Could you check a few things on this drawing? It's one solid part, dimensions in mm from its lowest x, y, z. A direction names the side the tool comes from. Round coordinates to 2 decimals unless told otherwise and drop trailing zeros. Loops run counter-clockwise (first coordinate to the right, second up) from the corner with the lowest first, then second, coordinate; pieces in that order, holes last. Notation, with made-up numbers: M -35.75,3 L -20.75,3 A23 ccw -20.75,34 Z; hole C 56,51.5 d6. An arc over 180 degrees is marked long. Write item = value, one per line. Start each with the question number.
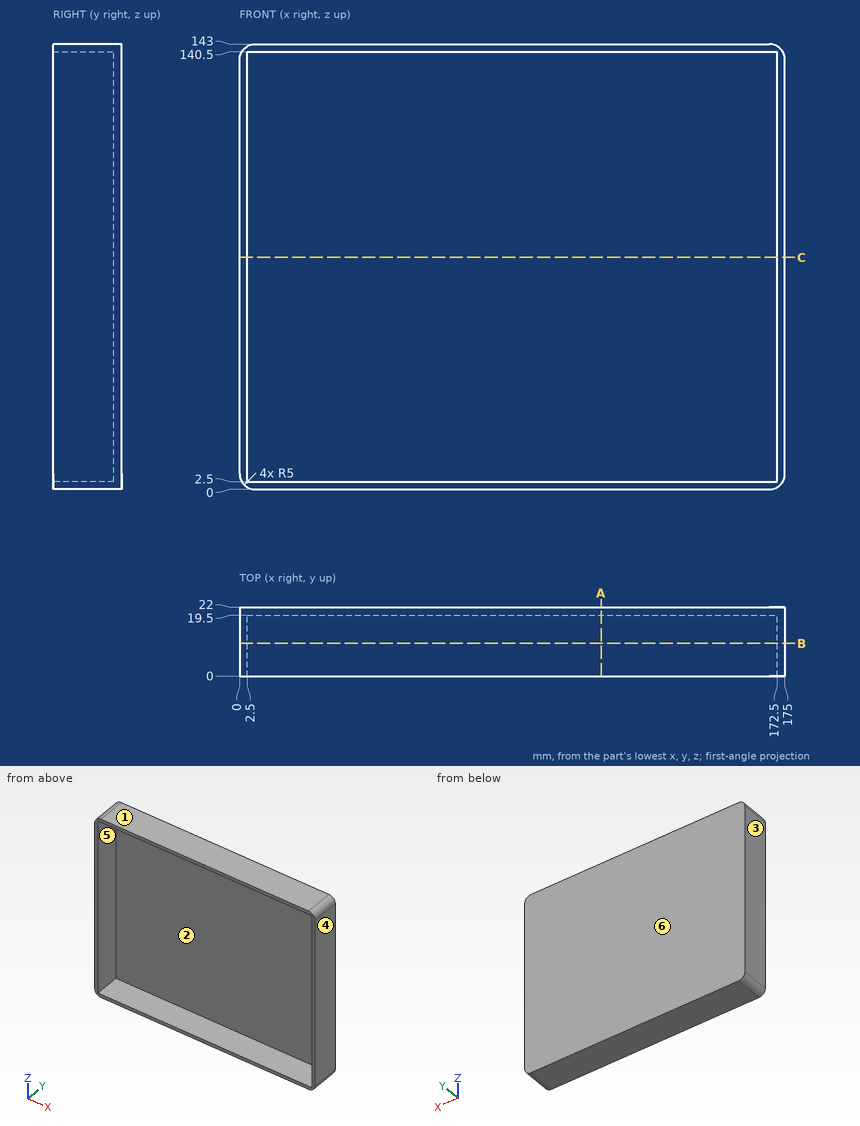
Item 1: We'd pull the mould along X, two halves only. Please class the marked faces 3, 4, 5 and 6: released by +X, released by -X, zero draft, split by the parting line, or undercut.
Item 2: I want a section at B-B, the plane y = 10.5. List the corners of the cut face in (x, z) for me.
Item 3: For the marked faces 1 and 2, which set-ups out of +Z, -Z, +X, -X, +Y, -Y let a thin tool reach every point of the face, with its end or its side?
Item 4: I want a section at A-A, the plane x = 116. List the corners of the cut face in (y, z) for me.
Item 5: Please list where these lines run through material, in increasing order: line 1 (Z direction, x = 27, y = 5); line 2 (X direction, y = 5.25, z = 45); line 3 (Y direction, x = 23.5, z = 125). Write a range as [from, to].
Item 6: Will this pin go through, and if not, where does the flat tip stop? pin 1 Ø10 at (x, z) = (107.5, 15) entering from -Y.
Item 7: I want a section at C-C, the plane z = 74.5. List the corners of the cut face in (x, y) for me.
Worked out:
q1.face_3 = released by -X
q1.face_4 = released by +X
q1.face_5 = undercut
q1.face_6 = zero draft
q2.outline = M 0,5 A5 ccw 5,0 L 170,0 A5 ccw 175,5 L 175,138 A5 ccw 170,143 L 5,143 A5 ccw 0,138 Z; hole M 2.5,2.5 L 172.5,2.5 L 172.5,140.5 L 2.5,140.5 Z
q3.face_1 = +Z, +X, -X, +Y, -Y
q3.face_2 = -Y
q4.outline = M 0,0 L 22,0 L 22,143 L 0,143 L 0,140.5 L 19.5,140.5 L 19.5,2.5 L 0,2.5 Z
q5.line_1 = [0, 2.5], [140.5, 143]
q5.line_2 = [0, 2.5], [172.5, 175]
q5.line_3 = [19.5, 22]
q6.pin_1 = 19.5
q7.outline = M 0,0 L 2.5,0 L 2.5,19.5 L 172.5,19.5 L 172.5,0 L 175,0 L 175,22 L 0,22 Z
